Input: part model. Units: mm. Frame: model coordinates. Coordinates: 2 decimals unless noted, no trailing zeros. Write each loop counter-clockwise with the first axis right and the second up, starting at its lowest first coordinate (ties: lowest second). Pieces come first, ordered by that corner, then holes. Notation, with made-up numbers: M -8.5,60.5 L 44.5,60.5 A18 ccw 44.5,69.5 Z; hole C 41,40.25 d1. An arc over 180 degrees is marked long. Use one line per item in the form item = value.
from build123d import *

# Parameters (mm, degrees)
F0_R     = 3.175
F1_DEPTH = 3.048
F2_DEPTH = 25.4


with BuildPart() as f1:
    # F0 (on Front) → F1 (new body)
    with BuildSketch(Plane.XZ):
        with BuildLine():
            ThreePointArc((-9.450293, 51.990625), (-0.596483, 41.293695), (9.525, 50.8))
            ThreePointArc((9.525, 50.8), (9.506305, 51.396483), (9.450293, 51.990625))
            ThreePointArc((9.450293, 51.990625), (0, 60.325), (-9.450293, 51.990625))
        make_face()
        with Locations((0, 50.8)):
            Circle(F0_R, mode=Mode.SUBTRACT)
        with BuildLine():
            ThreePointArc((9.525, -63.5), (-0.476848, -53.986944), (-9.477255, -64.4525))
            ThreePointArc((-9.477255, -64.4525), (-6.262383, -70.67692), (0.340179, -73.018923))
            ThreePointArc((0.340179, -73.018923), (6.854408, -70.113827), (9.525, -63.5))
        make_face()
        with Locations((0, -63.5)):
            Circle(F0_R, mode=Mode.SUBTRACT)
        with BuildLine():
            ThreePointArc((44.733482, -55.567564), (36.5125, -63.5), (44.733482, -71.432436))
            ThreePointArc((44.733482, -71.432436), (50.162007, -69.011523), (52.3875, -63.5))
            ThreePointArc((52.3875, -63.5), (50.162007, -57.988477), (44.733482, -55.567564))
        make_face()
        with Locations((44.45, -63.5)):
            Circle(F0_R, mode=Mode.SUBTRACT)
        with BuildLine():
            ThreePointArc((9.450293, 51.990625), (9.506305, 51.396483), (9.525, 50.8))
            ThreePointArc((9.525, 50.8), (-0.596483, 41.293695), (-9.450293, 51.990625))
            Line((-9.450293, 51.990625), (-15.750488, 1.984375))
            ThreePointArc((-15.750488, 1.984375), (0, 15.875), (15.750488, 1.984375))
            Line((15.750488, 1.984375), (9.450293, 51.990625))
        make_face()
        with Locations((-3.175, 35.60644)):
            Circle(F0_R, mode=Mode.SUBTRACT)
        with BuildLine():
            ThreePointArc((15.875, 0), (15.843841, 0.994139), (15.750488, 1.984375))
            ThreePointArc((15.750488, 1.984375), (0, 15.875), (-15.750488, 1.984375))
            ThreePointArc((-15.750488, 1.984375), (-15.873744, 0.199705), (-15.795426, -1.5875))
            ThreePointArc((-15.795426, -1.5875), (0, -15.875), (15.795426, -1.5875))
            ThreePointArc((15.795426, -1.5875), (15.855094, -0.794747), (15.875, 0))
        make_face()
        Circle(F0_R, mode=Mode.SUBTRACT)
        with BuildLine():
            ThreePointArc((15.795426, -1.5875), (0, -15.875), (-15.795426, -1.5875))
            Line((-15.795426, -1.5875), (-9.477255, -64.4525))
            ThreePointArc((-9.477255, -64.4525), (-0.476848, -53.986944), (9.525, -63.5))
            ThreePointArc((9.525, -63.5), (6.854408, -70.113827), (0.340179, -73.018923))
            Line((0.340179, -73.018923), (44.733482, -71.432436))
            ThreePointArc((44.733482, -71.432436), (36.5125, -63.5), (44.733482, -55.567564))
            Line((44.733482, -55.567564), (18.9676, -54.646766))
            ThreePointArc((18.9676, -54.646766), (13.2612, -51.928641), (11.341187, -45.906618))
            Line((11.341187, -45.906618), (15.795426, -1.5875))
        make_face()
    extrude(amount=F1_DEPTH)

    # F0 (on Front) → F2 (join)
    with BuildSketch(Plane.XZ):
        with BuildLine():
            ThreePointArc((-9.450293, 51.990625), (-0.596483, 41.293695), (9.525, 50.8))
            ThreePointArc((9.525, 50.8), (9.506305, 51.396483), (9.450293, 51.990625))
            ThreePointArc((9.450293, 51.990625), (0, 60.325), (-9.450293, 51.990625))
        make_face()
        with Locations((0, 50.8)):
            Circle(F0_R, mode=Mode.SUBTRACT)
        with BuildLine():
            ThreePointArc((9.450293, 51.990625), (9.506305, 51.396483), (9.525, 50.8))
            ThreePointArc((9.525, 50.8), (-0.596483, 41.293695), (-9.450293, 51.990625))
            Line((-9.450293, 51.990625), (-15.750488, 1.984375))
            ThreePointArc((-15.750488, 1.984375), (0, 15.875), (15.750488, 1.984375))
            Line((15.750488, 1.984375), (9.450293, 51.990625))
        make_face()
        with Locations((-3.175, 35.60644)):
            Circle(F0_R, mode=Mode.SUBTRACT)
        with BuildLine():
            ThreePointArc((15.875, 0), (15.843841, 0.994139), (15.750488, 1.984375))
            ThreePointArc((15.750488, 1.984375), (0, 15.875), (-15.750488, 1.984375))
            ThreePointArc((-15.750488, 1.984375), (-15.873744, 0.199705), (-15.795426, -1.5875))
            ThreePointArc((-15.795426, -1.5875), (0, -15.875), (15.795426, -1.5875))
            ThreePointArc((15.795426, -1.5875), (15.855094, -0.794747), (15.875, 0))
        make_face()
        Circle(F0_R, mode=Mode.SUBTRACT)
        with BuildLine():
            ThreePointArc((15.795426, -1.5875), (0, -15.875), (-15.795426, -1.5875))
            Line((-15.795426, -1.5875), (-9.477255, -64.4525))
            ThreePointArc((-9.477255, -64.4525), (-0.476848, -53.986944), (9.525, -63.5))
            ThreePointArc((9.525, -63.5), (6.854408, -70.113827), (0.340179, -73.018923))
            Line((0.340179, -73.018923), (44.733482, -71.432436))
            ThreePointArc((44.733482, -71.432436), (36.5125, -63.5), (44.733482, -55.567564))
            Line((44.733482, -55.567564), (18.9676, -54.646766))
            ThreePointArc((18.9676, -54.646766), (13.2612, -51.928641), (11.341187, -45.906618))
            Line((11.341187, -45.906618), (15.795426, -1.5875))
        make_face()
        with BuildLine():
            ThreePointArc((9.525, -63.5), (-0.476848, -53.986944), (-9.477255, -64.4525))
            ThreePointArc((-9.477255, -64.4525), (-6.262383, -70.67692), (0.340179, -73.018923))
            ThreePointArc((0.340179, -73.018923), (6.854408, -70.113827), (9.525, -63.5))
        make_face()
        with Locations((0, -63.5)):
            Circle(F0_R, mode=Mode.SUBTRACT)
        with BuildLine():
            ThreePointArc((44.733482, -55.567564), (36.5125, -63.5), (44.733482, -71.432436))
            ThreePointArc((44.733482, -71.432436), (50.162007, -69.011523), (52.3875, -63.5))
            ThreePointArc((52.3875, -63.5), (50.162007, -57.988477), (44.733482, -55.567564))
        make_face()
        with Locations((44.45, -63.5)):
            Circle(F0_R, mode=Mode.SUBTRACT)
    extrude(amount=F2_DEPTH)


solid = f1.part
(1) Pull-direction query (Z, two-part tool) for faces 1 (the flat face through (12.644, -12.522, 26.637)), 2 (the flat face through (13.537, -12.522, -24.057)), 3 (the cylindrical face through (-6.34, -12.52, -70.61)); classes: pulls with the +Z half, pulls with the -Z half, needs draft (parallel to the pull), parting line crosses it, or undercut.
Computed:
face_1 = pulls with the +Z half
face_2 = undercut
face_3 = pulls with the -Z half
(2) Section query C-C on z = -33. Return the cut outline in (x, y), plus the area to 3 significant figures.
Computed:
outline = M -12.64,-25.4 L 12.64,-25.4 L 12.64,0 L -12.64,0 Z
area = 642 mm^2
(3) Line query: probe 1 along X at (y, z) = (-6.75, 38); probe 2 along Z at (x, y) = (46, -14.5); probe 3 along Z at (x, y) = (42, -20.25). Output: solid intervals per line, ascending.
Computed:
probe_1 = -11.21 to -5.26, -1.09 to 11.21
probe_2 = -71.28 to -66.27, -60.73 to -55.72
probe_3 = -71.53 to -65.52, -61.48 to -55.47
(4) Section query D-D on x = 21. Return the cut outline in (y, z), plus the area to 3 significant figures.
Computed:
outline = M -25.4,-72.28 L 0,-72.28 L 0,-54.72 L -25.4,-54.72 Z
area = 446 mm^2
(5) Section query B-B on y = -16.5. State how many separate pieces and enclosed holes the cut face has, plus the area to 3 significant figures.
Computed:
separate_pieces = 1
enclosed_holes = 5
area = 3,770 mm^2
(6) Section query A-A on x = -1.5. Return the cut outline in (y, z), plus the area to 3 significant figures.
Computed:
outline = M -25.4,-72.91 L 0,-72.91 L 0,-66.3 L -25.4,-66.3 Z; M -25.4,-60.7 L 0,-60.7 L 0,-2.8 L -25.4,-2.8 Z; M -25.4,2.8 L 0,2.8 L 0,32.91 L -25.4,32.91 Z; M -25.4,38.3 L 0,38.3 L 0,48 L -25.4,48 Z; M -25.4,53.6 L 0,53.6 L 0,60.21 L -25.4,60.21 Z
area = 2,820 mm^2
(7) First-contact query: pin 1 Ø8 at (x, y) = (44.5, -6) entering from +Z; pin 2 Ø5.5 at (x, z) = (44.45, -63.5) entering from -Y; pin 3 Ø3 at (y, z) = (-19, 18) entering from +X; pin 4 Ø1.5 at (y, z) = (-7.5, -43.5) entering from +X. Flat tips, straight axial feed; report the tip coordinate or a pass-through.
Computed:
pin_1 = -55.42
pin_2 = through
pin_3 = 13.92
pin_4 = 11.66
